The drawing under review shows one solid part. Ordinate dimensions are in mm from its lowest x, y, z. Coordinates: 2 decimals unless noted, no trailing zeros. Write each loop counter-clockwise with the first axis right and the second up, starting at its lowest first coordinate (ties: lowest second). Pieces come first, ordered by that corner, then holes. Notation, with made-up numbers: (-13.75, 75) -> (28.25, 75) arc R10 cw to (28.25, 94) -> close; hole circle Ø1 at (65.25, 33.5). An arc over 180 degrees is marked (long way). One line per question, with ' | ' between items. Start each with the question number.
Q1. Add section B-B on x = 200. State the section outline as (y, z) points.
Q2. For P1, Ø8, axis at y = 12.5, z = 119.5, coming from the -X side; P2, Ø6, axis at x = 395, y = 10, coming from the -Z side; P3, Ø6, axis at x = 30, z = 26.25, coming from the -Y side; P4, Ø7.5, axis at y = 11, z = 257, coming from the +X side, all flat-tipped, find the tip position at first contact; note any pin that passes through.
Q3. Add section A-A on z = 40. State the section outline as (x, y) points.
Q4. Add section C-C on y = 6. State the section outline as (x, z) points, and give its area (3 significant figures).
Q5. Wall thickness on probe 1 along Z at (x, y) = (370, 4); probe 2 along X at (y, z) = (11.75, 26.25); probe 3 along X at (y, z) = (1.5, 325): over which ranges is each line inside the solid? List them lowest first.
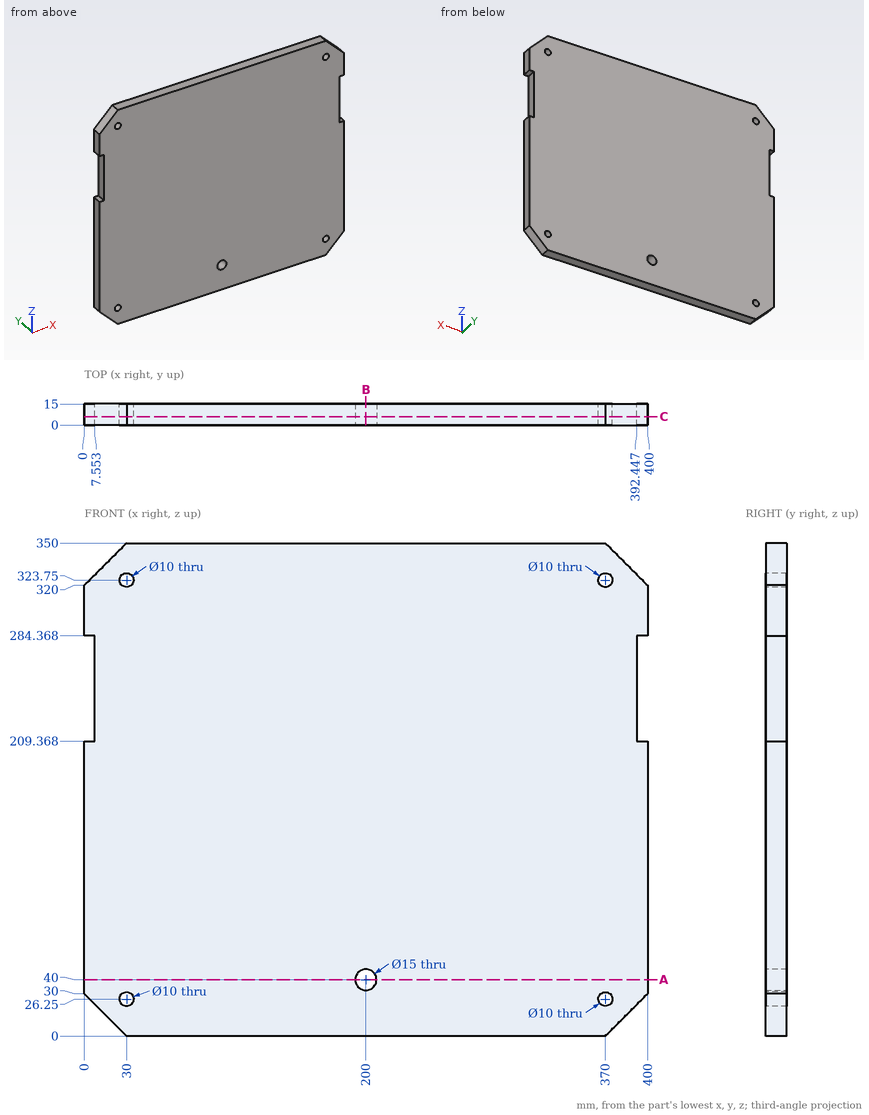
Output values:
1) outline: (0, 0) -> (15, 0) -> (15, 32.5) -> (0, 32.5) -> close; (0, 47.5) -> (15, 47.5) -> (15, 350) -> (0, 350) -> close
2) P1: stops at x = 0 | P2: stops at z = 22 | P3: passes through | P4: stops at x = 392.45
3) outline: (0, 0) -> (192.5, 0) -> (192.5, 15) -> (0, 15) -> close; (207.5, 0) -> (400, 0) -> (400, 15) -> (207.5, 15) -> close
4) outline: (0, 30) -> (30, 0) -> (370, 0) -> (400, 30) -> (400, 209.37) -> (392.45, 209.37) -> (392.45, 284.37) -> (400, 284.37) -> (400, 320) -> (370, 350) -> (30, 350) -> (0, 320) -> (0, 284.37) -> (7.55, 284.37) -> (7.55, 209.37) -> (0, 209.37) -> close; hole circle Ø10 at (30, 26.25); hole circle Ø10 at (30, 323.75); hole circle Ø15 at (200, 40); hole circle Ø10 at (370, 26.25); hole circle Ø10 at (370, 323.75) | area: 137,000 mm2
5) probe 1: z = 0 to 21.25, 31.25 to 318.75, 328.75 to 350 | probe 2: x = 3.75 to 25, 35 to 365, 375 to 396.25 | probe 3: x = 5 to 25.16, 34.84 to 365.16, 374.84 to 395
